```python
from build123d import *

# Parameters (mm, degrees)
SKETCH1_R           = 14.5
BOSS_EXTRUDE1_DEPTH = 147
SKETCH3_R           = 18
BOSS_EXTRUDE2_DEPTH = 17.5
BOSS_EXTRUDE3_START = 17.5
SKETCH4_R           = 18
BOSS_EXTRUDE3_DEPTH = 17.5
SKETCH5_R           = 4
BOSS_EXTRUDE4_DEPTH = 35
SKETCH2_R           = 11.5
CUT_EXTRUDE1_DEPTH  = 147


with BuildPart() as part:
    # Sketch1 → Boss-Extrude1 (new body)
    with BuildSketch(Plane.XY):
        Circle(SKETCH1_R)
    extrude(amount=BOSS_EXTRUDE1_DEPTH)

    # Sketch3 → Boss-Extrude2 (add)
    with BuildSketch(Plane(origin=(0, 0, 0), x_dir=(0, 0, -1), z_dir=(1, 0, 0))):
        with Locations(Location((-73.5, 7.25, 0), (0, 0, 156.248053974))):
            Circle(SKETCH3_R)
    extrude(amount=BOSS_EXTRUDE2_DEPTH)

    # Sketch4 → Boss-Extrude3 (add)
    with BuildSketch(Plane.ZY.offset(BOSS_EXTRUDE3_START)):
        with Locations((73.5, 7.25)):
            Circle(SKETCH4_R)
    extrude(amount=-BOSS_EXTRUDE3_DEPTH)

    # Sketch5 → Boss-Extrude4 (add)
    with BuildSketch(Plane(origin=(17.5, 0, 0), x_dir=(0, 0, -1), z_dir=(1, 0, 0))):
        with Locations((-60.288298956, 20.461701044)):
            Circle(SKETCH5_R)
        with Locations((-86.711701044, 20.461701044)):
            Circle(SKETCH5_R)
        with Locations((-60.288298956, -5.961701044)):
            Circle(SKETCH5_R)
        with Locations((-86.711701044, -5.961701044)):
            Circle(SKETCH5_R)
    extrude(amount=-BOSS_EXTRUDE4_DEPTH)

    # Sketch2 → Cut-Extrude1 (cut)
    with BuildSketch(Plane.XY.offset(147)):
        Circle(SKETCH2_R)
    extrude(amount=-CUT_EXTRUDE1_DEPTH, mode=Mode.SUBTRACT)


solid = part.part
```
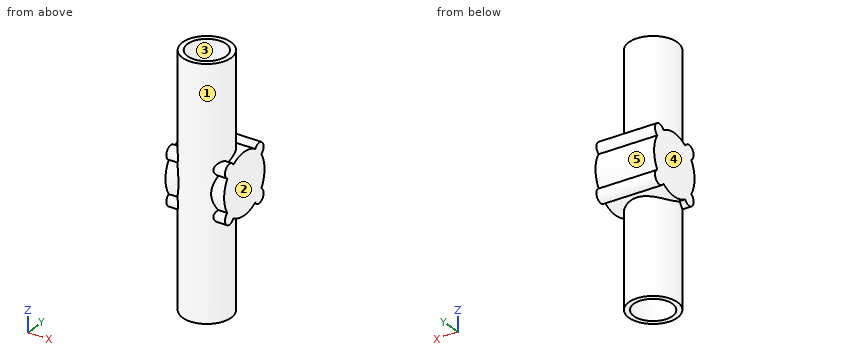
Build history of the part. All positions in model axes, mm. Face numbers are marked on the shaded views. A direction names the side the tool comes from. Round coordinates to 2 decimals unless told otherwise and drop trailing zeros. Loops run counter-clockwise (first coordinate to the right, second up) from the corner with the lowest first, then second, coordinate; pieces in that order, holes last.
Item 1: Which spindle directions (+Z, -Z, +X, -X, +Y, -Y) get a long thin tool onto all of the face, cutting with end or side? Do the marked faces 1 and 2. Say none if no direction does.
Item 2: Pin check, flat tips, straight feed: P1, Ø10, axis at y = 4, z = 128.5, coming from the +X side; P2, Ø2, axis at x = 0, y = 10, coming from the -Z side; P3, Ø5, axis at x = -13.5, z = 87, coming from the -Y side; P4, Ø1, axis at x = -9.5, z = 57.5, coming from the -Y side. Stop position of each tip, or through.
Item 3: Saw through at A-A (x = -2). List the corners of the cut face in (y, z).
Item 4: Drill centre lines: line 1 along Y through (x, z) = (0, 52.5); line 2 along Y through (x, z) = (3.5, 57); line 3 along Y through (x, z) = (-3.5, 92.5). Where is each one in solid material? Low to high.
Item 5: Two-plate mould, pull along Y, no slides. Class the marked faces 3, 4 and 5: released by +Y, released by -Y, zero draft, split by the parting line, or undercut.
Item 6: Saw through at C-C (z = 115). List the corners of the cut face in (x, y), then the cut area to 3 significant figures.
Item 7: Saw through at D-D (y = 8). List the corners of the cut face in (x, z), then the cut area to 3 significant figures.
Item 8: Saw through at B-B (y = 0). List the corners of the cut face in (x, z), then the cut area to 3 significant figures.
Worked answers:
1. face 1: none
1. face 2: +Z, -Z, +X, +Y, -Y
2. P1: stops at x = 14.5
2. P2: passes through
2. P3: stops at y = -9.96
2. P4: stops at y = -11.37
3. outline: (-14.36, 0) - (-11.32, 0) - (-11.32, 147) - (-14.36, 147) - close; (11.32, 0) - (14.36, 0) - (14.36, 56.96) arc R18 ccw to (16.96, 58.35) arc R4 ccw (long way) to (22.4, 63.79) arc R18 ccw to (22.4, 83.21) arc R4 ccw (long way) to (16.96, 88.65) arc R18 ccw to (14.36, 90.04) - (14.36, 147) - (11.32, 147) - close
4. line 1: y = -14.5 to -11.5, 11.5 to 14.5
4. line 2: y = -14.07 to -10.95, 10.95 to 14.44, 18.18 to 22.74
4. line 3: y = -14.07 to -10.95, 10.95 to 14.07
5. face 3: undercut
5. face 4: zero draft
5. face 5: released by +Y
6. outline: circle Ø29 at (0, 0); hole circle Ø23 at (0, 0)
6. area: 245 mm2
7. outline: (-17.5, 55.52) - (-12.09, 55.52) - (-12.09, 0) - (-8.26, 0) - (-8.26, 147) - (-12.09, 147) - (-12.09, 91.48) - (-17.5, 91.48) - close; (8.26, 0) - (12.09, 0) - (12.09, 55.52) - (17.5, 55.52) - (17.5, 91.48) - (12.09, 91.48) - (12.09, 147) - (8.26, 147) - close
7. area: 1,520 mm2
8. outline: (-17.5, 57.02) - (-14.5, 57.02) - (-14.5, 0) - (-11.5, 0) - (-11.5, 147) - (-14.5, 147) - (-14.5, 89.98) - (-17.5, 89.98) - close; (11.5, 0) - (14.5, 0) - (14.5, 57.02) - (17.5, 57.02) - (17.5, 89.98) - (14.5, 89.98) - (14.5, 147) - (11.5, 147) - close
8. area: 1,080 mm2
